Verification items for the finished model (mm, model axes). A direction names the side the tool comes from. Round coordinates to 2 decimals unless told otherwise and drop trailing zeros. Order: outer loops, then holes, each group sorted by start corner. A loop starts at its lowest first (then second) coordinate and runs counter-clockwise, first axis right, second up. Notation, with made-up numbers: (-20.75, -22) -> (35.25, -22) arc R32 ccw to (35.25, 13) -> close; hole circle Ø11 at (26.5, 55.25). An arc over 180 degrees is marked (long way). Put each result on its own line as item: value.
```python
from build123d import *

# Parameters (mm, degrees)
F1_DEPTH = 70
F2_SIZE2 = 11.1961524227
F2_SIZE  = 3
F4_T     = -1
F5_DEPTH = 1
F6_SIZE  = 0.3


with BuildPart() as f1:
    # F0 (on Top) → F1 (new body)
    with BuildSketch(Plane.XY):
        Polygon((30, 10), (25, 15), (-25, 15), (-30, 10), (-30, -10), (-25, -15), (25, -15), (30, -10), align=None)
        Polygon((-22.9289321881, 10), (22.9289321881, 10), (25, 7.9289321881), (25, -7.9289321881), (22.9289321881, -10), (-22.9289321881, -10), (-25, -7.9289321881), (-25, 7.9289321881), align=None, mode=Mode.SUBTRACT)
    extrude(amount=F1_DEPTH)

    # F2
    f2_edges = [f1.edges().sort_by_distance(p)[0] for p in [
        (-30, 0, 70),
        (-27.5, -12.5, 70),
        (0, -15, 70),
        (27.5, -12.5, 70),
        (30, 0, 70),
        (27.5, 12.5, 70),
        (0, 15, 70),
        (-27.5, 12.5, 70),
    ]]
    f2_side = f1.faces().sort_by_distance((27.025658, 12.025658, 70))[0]
    chamfer(f2_edges, length=F2_SIZE, length2=F2_SIZE2, reference=f2_side)

    # F3: F1 across face


with BuildPart() as f1_1:
    add(f1.part)
    add(f1.part.mirror(Plane(origin=(0, 0, 0), x_dir=(1, 0, 0), z_dir=(0, 0, -1))))

    # F4
    f4_openings = [f1_1.faces().sort_by_distance(p)[0] for p in [
        (-25, 0, 0),
        (-23.964466, 8.964466, 0),
        (0, 10, 0),
        (23.964466, 8.964466, 0),
        (25, 0, 0),
        (0, -10, 0),
        (-23.964466, -8.964466, 0),
        (23.964466, -8.964466, 0),
    ]]
    offset(amount=F4_T, openings=f4_openings)

    # F5 (add): a face of the model
    f5_faces = [f1_1.faces().sort_by_distance(p)[0] for p in [
        (-26.4090685319, 0, -70),
    ]]
    extrude(f5_faces, amount=F5_DEPTH)

    # F6
    f6_edges = [f1_1.edges().sort_by_distance(p)[0] for p in [
        (-27, 0, -71),
        (-25.37868, 10.37868, -71),
        (-25.37868, -10.37868, -71),
        (0, 12, -71),
        (0, -12, -71),
        (25.37868, 10.37868, -71),
        (25.37868, -10.37868, -71),
        (27, 0, -71),
        (0, 10, -71),
        (23.964466, 8.964466, -71),
        (25, 0, -71),
        (23.964466, -8.964466, -71),
        (0, -10, -71),
        (-23.964466, -8.964466, -71),
        (-25, 0, -71),
        (-23.964466, 8.964466, -71),
    ]]
    chamfer(f6_edges, length=F6_SIZE)


solid = f1_1.part
```
Item 1: Tool access check on faces 4 (the face through (25.4, 10.36, -70.35)), 5 (the face through (25.8, -10.86, 63.76)), 6 (the face through (-24.053, -9.085, -70.848)). Record the directions out of +Z, -Z, +X, -X, +Y, -Y that give a thin tool (end or side, any length) a straight path to the whole face; none if there is none.
Geometry check:
face 4: -Z, +X, +Y
face 5: none
face 6: -Z
Item 2: Depth check by flat-ended pin: pin 1 Ø1.9 at (y, z) = (-1.5, -69.5) entering from -X; pin 2 Ø0.5 at (y, z) = (0, 69.5) entering from -X; pin 3 Ø1.1 at (x, z) = (-6.5, 69.5) entering from -Y; pin 4 Ø6.5 at (x, y) = (-9.5, -4) entering from +Z. Enter the tip coordinate at first touch or a pass-through.
Geometry check:
pin 1: x = -27.39
pin 2: x = -27.2
pin 3: y = -12.28
pin 4: through
Item 3: Sectioned sample at C-C, the plane z = -20. Record the boundary of the cut face in (x, y).
Geometry check:
outline: (-30, -10) -> (-25, -15) -> (25, -15) -> (30, -10) -> (30, 10) -> (25, 15) -> (-25, 15) -> (-30, 10) -> close; hole (-29, -9.59) -> (-24.59, -14) -> (24.59, -14) -> (29, -9.59) -> (29, 9.59) -> (24.59, 14) -> (-24.59, 14) -> (-29, 9.59) -> close
Item 4: Release check for a two-part mould opening along Z. For faces 1 (the face through (0.35, 13.52, -64.32)), 2 (the face through (0.35, 13.52, 64.32)), 3 (the face through (-27.636, 0.134, 63.764)) record: pulls with the +Z half, pulls with the -Z half, needs draft (parallel to the pull), parting line crosses it, or undercut.
Geometry check:
face 1: pulls with the -Z half
face 2: pulls with the +Z half
face 3: undercut
Item 5: Material ranges on line 1 along Z through (x, y) = (-25, 8.5); line 2 along X through (y, z) = (-9.25, 24); line 3 along Y through (x, z) = (-18.5, 48), recorded low to high.
Geometry check:
line 1: -71 to -69, 69 to 70
line 2: -30 to -29, 29 to 30
line 3: -15 to -14, 14 to 15
